For this review, use the dimensioned drawing (mm, ordinates from the lowest corner) and the shaded views. Round coordinates to 2 decimals unless told otherwise and drop trailing zeros. Loops run counter-clockwise (first coordinate to the right, second up) from the corner with the lowest first, then second, coordinate; pieces in that order, holes last. Notation, with made-up numbers: (70, 29.25) - (121, 29.25) arc R17 ccw to (121, 51.25) - close; hole circle Ø1 at (33, 60). An arc over 180 degrees is marked (long way). Use one line per item in the form item = value. Start each with the question number.
(1) For pin 1 (0.6 mm diameter, centred on x = 11, y = 0.5, fed in from -Z); pin 2 (0.6 mm diameter, centred on y = 1, z = 33, fed in from +X); pin 3 (0.6 mm diameter, centred on x = 11.5, y = 0.5, fed in from +Z), all flat-tipped, find the tip position at first contact; note any pin that passes through.
(2) Wall thickness on probe 1 along Z at (x, y) = (11.5, 1): over which ranges is the line inside the solid? List them lowest first. Write a range as [from, to].
(3) We need section A-A, the plane y = 0.6. Write out the cut boundary in (x, z).
(4) We need section B-B, the plane x = 11. Write out the cut boundary in (y, z).
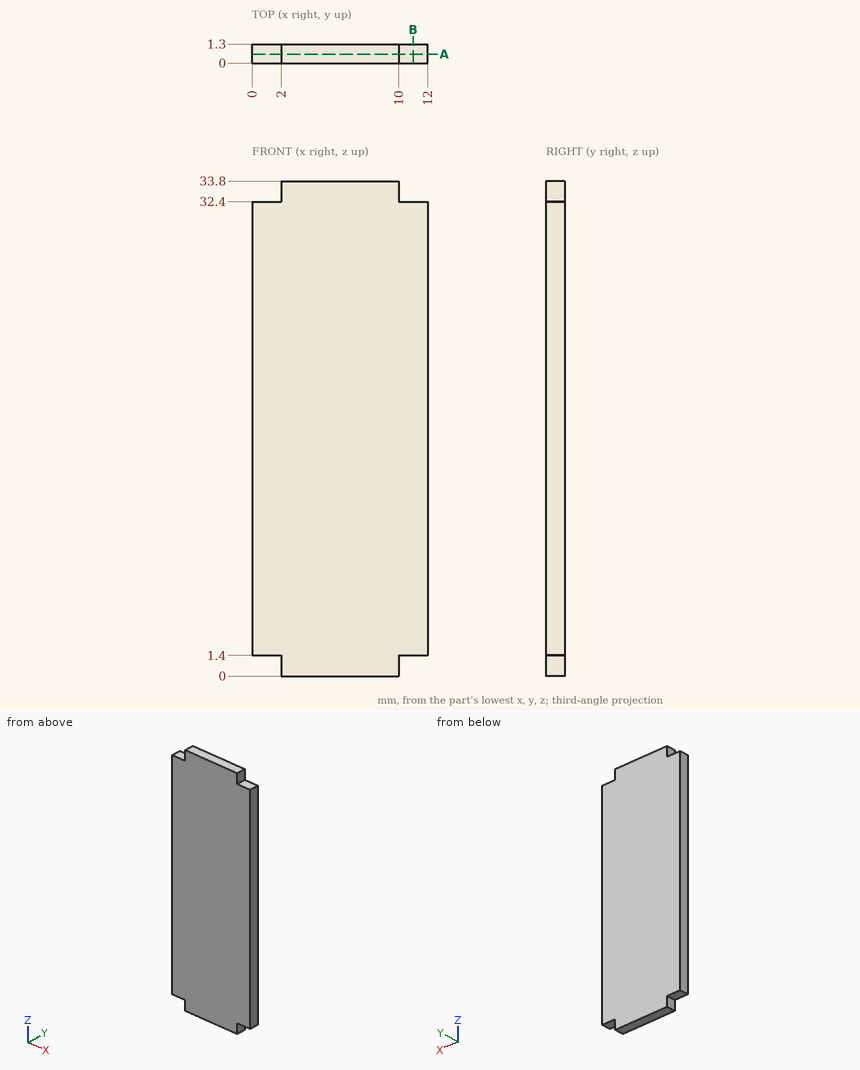
Data:
q1.pin_1 = 1.4
q1.pin_2 = 10
q1.pin_3 = 32.4
q2.probe_1 = [1.4, 32.4]
q3.outline = (0, 1.4) - (2, 1.4) - (2, 0) - (10, 0) - (10, 1.4) - (12, 1.4) - (12, 32.4) - (10, 32.4) - (10, 33.8) - (2, 33.8) - (2, 32.4) - (0, 32.4) - close
q4.outline = (0, 1.4) - (1.3, 1.4) - (1.3, 32.4) - (0, 32.4) - close
